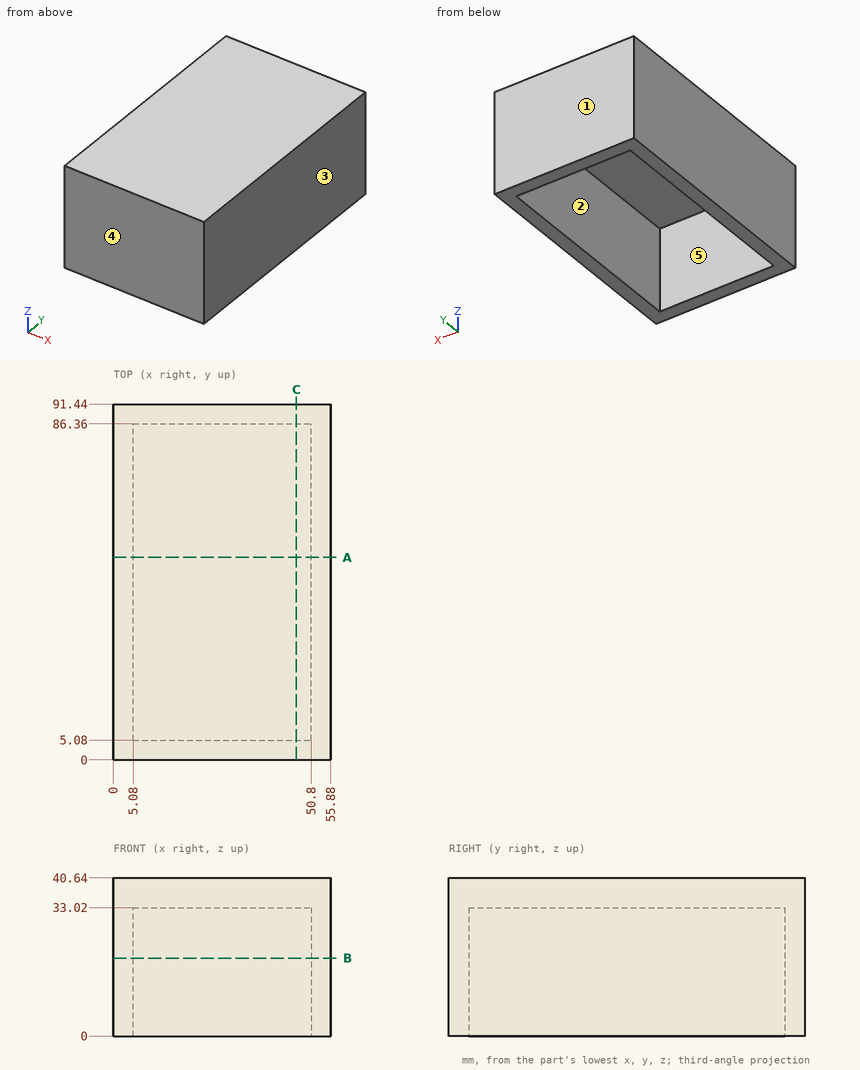
Answer from the drawing. Dimensions are ordinates in mm from the lowest x, y and z of the part. A direction names the side the tool comes from. Round coordinates to 2 decimals unless told otherwise and drop trailing zeros. Write each loop counter-clockwise with the first axis right and the second up, starting at its lowest first coordinate (ties: lowest second). Pieces come first, ordered by that corner, then holes. Notation, with made-up numbers: (31.5, 82.25) -> (71.5, 82.25) arc R21 cw to (71.5, 102.25) -> close; hole circle Ø6 at (-25, -12). An arc over 180 degrees is marked (long way). Write each question's results on one line, items separated by ' | '.
1) The part is cut by section C-C (x = 47). Write down the section's boundary in (y, z).
Findings:
outline: (0, 0) -> (5.08, 0) -> (5.08, 33.02) -> (86.36, 33.02) -> (86.36, 0) -> (91.44, 0) -> (91.44, 40.64) -> (0, 40.64) -> close
2) The part is cut by section B-B (z = 20). Write down the section's boundary in (x, y), and give its area (3 significant figures).
Findings:
outline: (0, 0) -> (55.88, 0) -> (55.88, 91.44) -> (0, 91.44) -> close; hole (5.08, 5.08) -> (50.8, 5.08) -> (50.8, 86.36) -> (5.08, 86.36) -> close | area: 1,390 mm²
3) A flat-ended cylindrical pin translates along its axis: pin 1 (4 mm diameter, centred on x = 12, y = 74, fed in from -Z). Find the tip coordinate at first contact, or state that the pin passes through.
Findings:
pin 1: stops at z = 33.02
4) The part is cut by section A-A (y = 52). Write down the section's boundary in (x, z), and give its area (3 significant figures).
Findings:
outline: (0, 0) -> (5.08, 0) -> (5.08, 33.02) -> (50.8, 33.02) -> (50.8, 0) -> (55.88, 0) -> (55.88, 40.64) -> (0, 40.64) -> close | area: 761 mm²
5) Which of the six approach directions +Z, -Z, +X, -X, +Y, -Y give full straight-line access (tool end or side, diameter ignored) to the marked faces 4 and 5?
Findings:
face 4: +Z, -Z, +X, -X, -Y | face 5: -Z
6) For a pull along Y with two mould halves and no side action, classify the marked faces 1, 2 and 3 as +Y half, -Y half, draft (parallel to the pull), parting line (faces both ways), or undercut.
Findings:
face 1: +Y half | face 2: undercut | face 3: draft
7) Consider line 1 along X through (y, z) = (8.5, 28); line 2 along Y through (x, z) = (33.5, 30); line 3 along Z through (x, y) = (48, 46.5). Determine where each line is inside the solid, lowest interval first. Write a range as [from, to].
Findings:
line 1: x = [0, 5.08], [50.8, 55.88] | line 2: y = [0, 5.08], [86.36, 91.44] | line 3: z = [33.02, 40.64]
